Part print with two shaded views. Sizes in mm from the minimum x, y, z corner. Coordinates: 2 decimals unless noted, no trailing zeros. Loops run counter-clockwise (first coordinate to the right, second up) from the corner with the lowest first, then second, coordinate; pieces in that order, holes last. Notation, with made-up numbers: (88.25, 43.25) -> (113.25, 43.25) arc R18 cw to (113.25, 77.25) -> close; hole circle Ø6 at (60.5, -9). An arc over 180 degrees is marked (long way). Write each question's results on one line, items separated by ' | '.
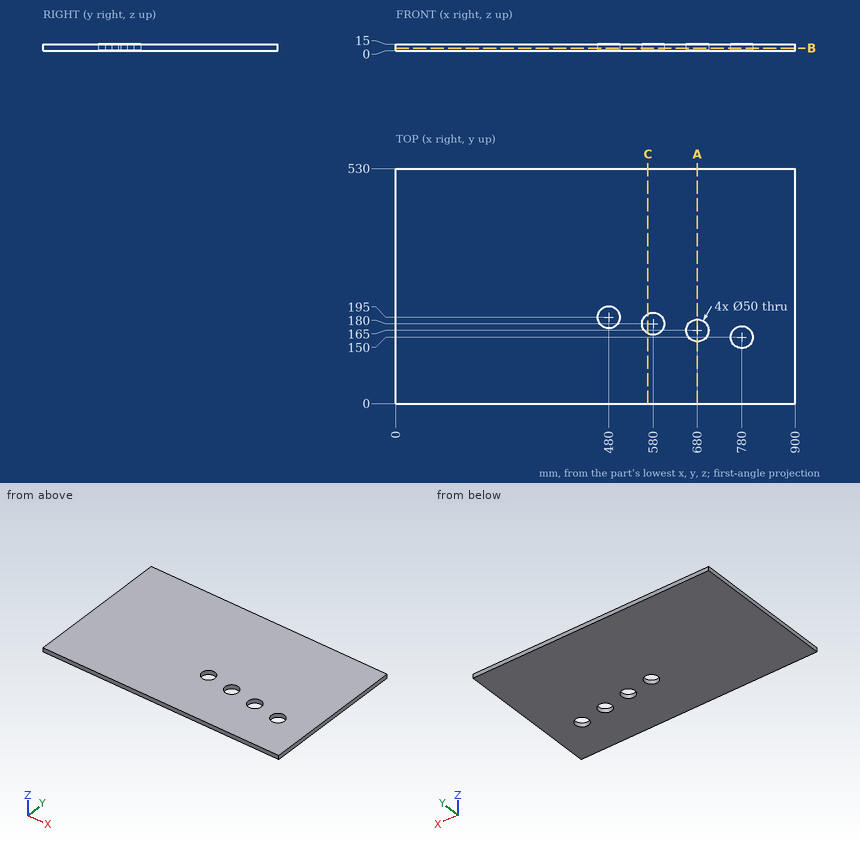
Q1. Cut at B-B on z = 5.5. Write the cut outline in (x, y), and give its area (3 significant figures).
Results are:
outline: (0, 0) -> (900, 0) -> (900, 530) -> (0, 530) -> close; hole circle Ø50 at (480, 195); hole circle Ø50 at (580, 180); hole circle Ø50 at (680, 165); hole circle Ø50 at (780, 150) | area: 469,000 mm^2
Q2. Cut at C-C on x = 568. Write the cut outline in (y, z).
Results are:
outline: (0, 0) -> (158.07, 0) -> (158.07, 15) -> (0, 15) -> close; (201.93, 0) -> (530, 0) -> (530, 15) -> (201.93, 15) -> close
Q3. Wall check: L1, parallel to Y at x = 580, z = 5; L2, parallel to Y at x = 780, z = 8.75; L3, parallel to X at y = 200.5, z = 7.25. Give the ranges that are in metal, low to high. Write a range as from..to.
Results are:
L1: 0..155, 205..530 | L2: 0..125, 175..530 | L3: 0..455.61, 504.39..565.69, 594.31..900
Q4. Drop a flat-ended pin along its axis: pin 1 (3 mm diameter, centred on x = 423.5, y = 182, fed in from -Z). Give the stop position or say it passes through.
Results are:
pin 1: z = 0
Q5. Cut at A-A on x = 680. Write the cut outline in (y, z), and give its area (3 significant figures).
Results are:
outline: (0, 0) -> (140, 0) -> (140, 15) -> (0, 15) -> close; (190, 0) -> (530, 0) -> (530, 15) -> (190, 15) -> close | area: 7,200 mm^2
